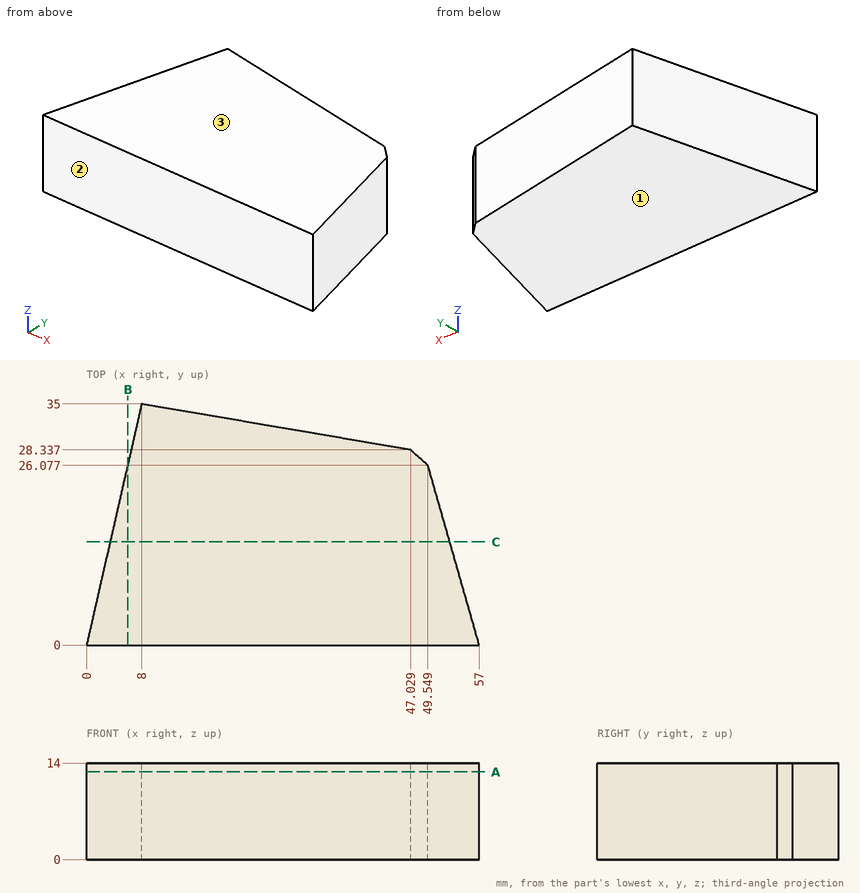
Geometry: see drawing. Coordinates: mm, zero at the bounding-box minimum. Give positions to 0.01 mm unless a question says otherwise; leave off trailing zeros. Loops run counter-clockwise (first coordinate to the right, second up) from the corner with the lowest first, then second, coordinate; pieces in that order, holes last. Notation, with made-up numbers: (50, -24.5) -> (100, -24.5) arc R35 ccw to (100, 12.5) -> close; hole circle Ø4 at (17.25, 67). An arc over 180 degrees is marked (long way). Put each result on its own line as item: value.
1. Pull-direction query (Z, two-part tool) for the marked faces 1, 2 and 3; classes: released by +Z, released by -Z, zero draft, split by the parting line, or undercut.
Taken from the geometry:
face 1: released by -Z
face 2: zero draft
face 3: released by +Z
2. Cut plane A-A (z = 12.75). Return the cut outline in (x, y), plus the area to 3 significant figures.
Taken from the geometry:
outline: (0, 0) -> (57, 0) -> (49.55, 26.08) -> (47.03, 28.34) -> (8, 35) -> close
area: 1,540 mm2
3. Cut plane C-C (y = 15). Return the cut outline in (x, z) (1 decimal), plus the area to 3 significant figures.
Taken from the geometry:
outline: (3.4, 0) -> (52.7, 0) -> (52.7, 14) -> (3.4, 14) -> close
area: 690 mm2
4. Ray query, line 1 along X through (y, z) = (17.5, 12.25); line 2 along X through (y, z) = (27.5, 3.25) (1 decimal); line 3 along Y through (x, z) = (38, 10.75). Return the intervals inside material, ascending. Write a range as [from, to].
Taken from the geometry:
line 1: x = [4, 52]
line 2: x = [6.3, 48]
line 3: y = [0, 29.88]
5. Pin query (flat end, axial travel): P1, Ø1.5, axis at y = 23.5, z = 7.5, coming from the -X side; P2, Ø1.5, axis at y = 29, z = 10, coming from the -X side; P3, Ø4, axis at x = 42.5, z = 5, coming from the +Y side. Return the tip coordinate at first contact, or that it passes through.
Taken from the geometry:
P1: stops at x = 5.2
P2: stops at x = 6.46
P3: stops at y = 29.45
6. Cut plane B-B (x = 6). Return the cut outline in (y, z).
Taken from the geometry:
outline: (0, 0) -> (26.25, 0) -> (26.25, 14) -> (0, 14) -> close
